Geometry: see drawing. Coordinates: mm, zero at the bounding-box minimum. Give positions to 0.01 mm unless a question says otherwise; leave off trailing zeros. Loops run counter-clockwise (first coordinate to the right, second up) from the corner with the lowest first, then second, coordinate; pieces in that order, holes last. Notation, with made-up numbers: (20.25, 72.5) -> (47.25, 72.5) arc R21 ccw to (47.25, 97.5) -> close; hole circle Ø10 at (36, 0). An arc over 180 degrees is marked (long way). Return JSON: item names as keys, results as strings. Group by question number.
(1) Cut plane A-A on x = 19. Return loops of the section in (y, z) (3 decimals), then the cut area to 4 significant figures.
(2) Ray query, line 1 (Y direction, x = 19, z = 0.55) (3 decimals); line 2 (X direction, y = 3.5, z = 0.85); line 3 (X direction, y = 5.75, z = 0.8). Return the intervals inside material, ascending. Write a range as from..to.
(3) Draft query along Y for the marked faces 1, 2, 3 and 4. Return one class per face: released by +Y, released by -Y, zero draft, split by the parting line, or undercut.
(4) Cut plane D-D on x = 4.75. Return loops of the section in (y, z).
(5) Cut plane B-B on y = 4. Return loops of the section in (x, z) (3 decimals), then the cut area to 4 significant figures.
(6) Cut plane C-C on z = 0.85. Return loops of the section in (x, y) (3 decimals), then the cut area to 3 significant figures.
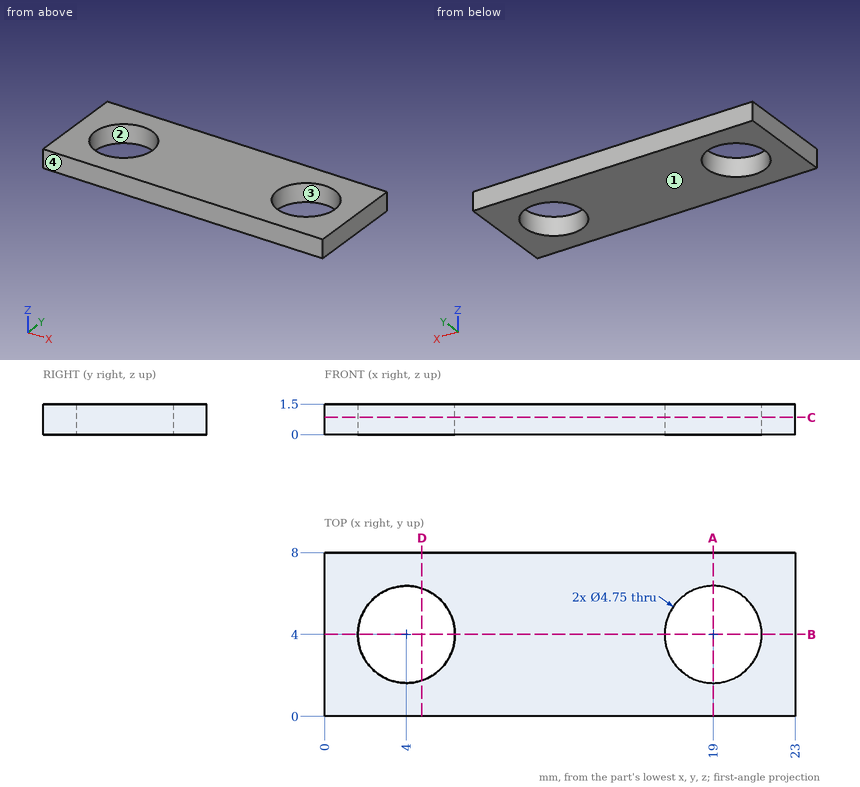
Answers:
{
 "1": {"outline": "(0, 0) -> (1.625, 0) -> (1.625, 1.5) -> (0, 1.5) -> close; (6.375, 0) -> (8, 0) -> (8, 1.5) -> (6.375, 1.5) -> close", "area": "4.875 mm²"},
 "2": {"line 1": "0..1.625, 6.375..8", "line 2": "0..1.68, 6.32..16.68, 21.32..23", "line 3": "0..2.39, 5.61..17.39, 20.61..23"},
 "3": {"face 1": "zero draft", "face 2": "undercut", "face 3": "undercut", "face 4": "released by -Y"},
 "4": {"outline": "(0, 0) -> (1.75, 0) -> (1.75, 1.5) -> (0, 1.5) -> close; (6.25, 0) -> (8, 0) -> (8, 1.5) -> (6.25, 1.5) -> close"},
 "5": {"outline": "(0, 0) -> (1.625, 0) -> (1.625, 1.5) -> (0, 1.5) -> close; (6.375, 0) -> (16.625, 0) -> (16.625, 1.5) -> (6.375, 1.5) -> close; (21.375, 0) -> (23, 0) -> (23, 1.5) -> (21.375, 1.5) -> close", "area": "20.25 mm²"},
 "6": {"outline": "(0, 0) -> (23, 0) -> (23, 8) -> (0, 8) -> close; hole circle Ø4.75 at (4, 4); hole circle Ø4.75 at (19, 4)", "area": "149 mm²"}
}
